Verification items for the finished model (mm, model axes). Round coordinates to 2 decimals unless told otherwise and drop trailing zeros. Order: outer loops, then holes, each group sorted by start corner. A loop starts at its lowest first (then second) coordinate and runs counter-clockwise, first axis right, second up. Notation, with made-up numbers: (-17, 14) -> (10, 14) arc R9 ccw to (10, 28) -> close; hole circle Ø11 at (-29, 60.25). An arc over 180 degrees is marked (long way). Put each result on its own line as item: value.
from build123d import *

# Parameters (mm, degrees)
F0_W     = 72.89
F0_H     = 53.72
F1_DEPTH = 2
F2_DEPTH = 1
F3_START = 1
F0_W_2   = 2.2
F0_H_2   = 12.58
F3_DEPTH = 1
F4_R     = 0.6


with BuildPart() as f1:
    # F0 (on Top) → F1 (new body)
    with BuildSketch(Plane.XY):
        with Locations((5.6164505921, 7.9296875)):
            Rectangle(F0_W, F0_H)
        Polygon((-21.5285494079, 30.8196875), (37.6814505921, 30.8196875), (37.6814505921, -11.7603125), (-21.5285494079, -11.7603125), (-21.5285494079, 13.2396875), (-23.7285494079, 13.2396875), (-23.7285494079, 25.8196875), (-21.5285494079, 25.8196875), align=None, mode=Mode.SUBTRACT)
        Polygon((37.6814505921, -11.7603125), (37.6814505921, 30.8196875), (-21.5285494079, 30.8196875), (-21.5285494079, 25.8196875), (-21.5285494079, 13.2396875), (-21.5285494079, -11.7603125), align=None)
        with BuildLine():
            ThreePointArc((-19.1285494079, 28.3196875), (-18.835656189, 29.0267942812), (-18.1285494079, 29.3196875))
            Line((-18.1285494079, 29.3196875), (35.1314505921, 29.3196875))
            ThreePointArc((35.1314505921, 29.3196875), (35.8385573733, 29.0267942812), (36.1314505921, 28.3196875))
            Line((36.1314505921, 28.3196875), (36.1314505921, -9.2603125))
            ThreePointArc((36.1314505921, -9.2603125), (35.8385573733, -9.9674192812), (35.1314505921, -10.2603125))
            Line((35.1314505921, -10.2603125), (-18.1285494079, -10.2603125))
            ThreePointArc((-18.1285494079, -10.2603125), (-18.835656189, -9.9674192812), (-19.1285494079, -9.2603125))
            Line((-19.1285494079, -9.2603125), (-19.1285494079, 28.3196875))
        make_face(mode=Mode.SUBTRACT)
    extrude(amount=F1_DEPTH)

    # F0 (on Top) → F2 (cut)
    with BuildSketch(Plane.XY):
        Polygon((37.6814505921, -11.7603125), (37.6814505921, 30.8196875), (-21.5285494079, 30.8196875), (-21.5285494079, 25.8196875), (-21.5285494079, 13.2396875), (-21.5285494079, -11.7603125), align=None)
        with BuildLine():
            ThreePointArc((-19.1285494079, 28.3196875), (-18.835656189, 29.0267942812), (-18.1285494079, 29.3196875))
            Line((-18.1285494079, 29.3196875), (35.1314505921, 29.3196875))
            ThreePointArc((35.1314505921, 29.3196875), (35.8385573733, 29.0267942812), (36.1314505921, 28.3196875))
            Line((36.1314505921, 28.3196875), (36.1314505921, -9.2603125))
            ThreePointArc((36.1314505921, -9.2603125), (35.8385573733, -9.9674192812), (35.1314505921, -10.2603125))
            Line((35.1314505921, -10.2603125), (-18.1285494079, -10.2603125))
            ThreePointArc((-18.1285494079, -10.2603125), (-18.835656189, -9.9674192812), (-19.1285494079, -9.2603125))
            Line((-19.1285494079, -9.2603125), (-19.1285494079, 28.3196875))
        make_face(mode=Mode.SUBTRACT)
    extrude(amount=F2_DEPTH, mode=Mode.SUBTRACT)

    # F0 (on Top) → F3 (join)
    with BuildSketch(Plane.XY.offset(F3_START)):
        with Locations((-22.6285494079, 19.5296875)):
            Rectangle(F0_W_2, F0_H_2)
    extrude(amount=F3_DEPTH)

    # F4
    f4_edges = [f1.edges().sort_by_distance(p)[0] for p in [
        (8.501451, 29.319688, 2),
        (-19.128549, 9.529688, 2),
        (8.501451, -10.260312, 2),
        (36.131451, 9.529688, 2),
    ]]
    fillet(f4_edges, radius=F4_R)


solid = f1.part
Item 1: Section check C-C on z = 0.4. Record the boundary of the cut face in (x, y).
Check sheet entries:
outline: (-30.83, -18.93) -> (42.06, -18.93) -> (42.06, 34.79) -> (-30.83, 34.79) -> close; hole (-23.73, 13.24) -> (-21.53, 13.24) -> (-21.53, -11.76) -> (37.68, -11.76) -> (37.68, 30.82) -> (-21.53, 30.82) -> (-21.53, 25.82) -> (-23.73, 25.82) -> close
Item 2: Section check B-B on x = 34. Record the boundary of the cut face in (y, z).
Check sheet entries:
outline: (-18.93, 0) -> (-11.76, 0) -> (-11.76, 1) -> (-10.26, 1) -> (-10.26, 1.4) arc R0.6 ccw to (-10.86, 2) -> (-18.93, 2) -> close; (29.32, 1) -> (30.82, 1) -> (30.82, 0) -> (34.79, 0) -> (34.79, 2) -> (29.92, 2) arc R0.6 ccw to (29.32, 1.4) -> close
Item 3: Release check for a two-part mould opening along X. For faces 1 (the flat face through (5, -16, 2)), 2 (the flat face through (-30.829, 8, 1)), 3 (the flat face through (5, 30, 1)) record: +X half, -X half, draft (parallel to the pull), parting line (faces both ways), or undercut.
Check sheet entries:
face 1: draft
face 2: -X half
face 3: undercut
Item 4: Material ranges on L1, parallel to Y at x = 9.5, z = 0.9; L2, parallel to X at y = 10.5, z = 0.9; L3, parallel to Y at x = 22, z = 1.05, recorded low to high. Write a range as [from, to].
Check sheet entries:
L1: y = [-18.93, -11.76], [30.82, 34.79]
L2: x = [-30.83, -21.53], [37.68, 42.06]
L3: y = [-18.93, -10.26], [29.32, 34.79]
Item 5: Section check A-A on y = 14. Record the boundary of the cut face in (x, z), then the cut area to 3 significant figures.
Check sheet entries:
outline: (-30.83, 0) -> (-23.73, 0) -> (-23.73, 1) -> (-19.13, 1) -> (-19.13, 1.4) arc R0.6 ccw to (-19.73, 2) -> (-30.83, 2) -> close; (36.13, 1) -> (37.68, 1) -> (37.68, 0) -> (42.06, 0) -> (42.06, 2) -> (36.73, 2) arc R0.6 ccw to (36.13, 1.4) -> close
area: 29.0 mm^2
